from build123d import *

# Parameters (mm, degrees)
F0_W         = 52.4178380828
F0_H         = 38.1
F1_DEPTH     = 152.4
F3_DEPTH     = 152.401
F5_DEPTH     = 12.7
F7_DEPTH     = 19.05
F8_W         = 5.08
F8_H         = 2.54
F9_DEPTH     = 52.4188380828
F10_R        = 2.54
F11_T1_DEPTH = 18.199261314


# Not quite as in the source:
# - a fillet or chamfer that OpenCascade refuses, or shapes differently, is made with other operations: its cross-section is extruded or revolved along the edge and cut away or added


with BuildPart() as f1:
    # F0 (on Right) → F1 (new body)
    with BuildSketch(Plane.YZ):
        Rectangle(F0_W, F0_H)
    extrude(amount=-F1_DEPTH)

    # F2 (on face) → F3 (cut, through all)
    with BuildSketch(Plane.YZ):
        with BuildLine():
            Line((6.6756140975, -19.05), (10.4856140975, -19.05))
            Line((10.4856140975, -19.05), (10.4856140975, -2.54))
            ThreePointArc((10.4856140975, -2.54), (10.1136397096, -1.6419743879), (9.2156140975, -1.27))
            Line((9.2156140975, -1.27), (-9.2156140975, -1.27))
            ThreePointArc((-9.2156140975, -1.27), (-10.0011773128, -1.5421070023), (-10.4501149349, -2.241826087))
            Line((-10.4501149349, -2.241826087), (-13.6443859025, -15.4667596303))
            Line((-13.6443859025, -15.4667596303), (-9.9408833902, -16.3612813694))
            Line((-9.9408833902, -16.3612813694), (-7.2160704876, -5.08))
            Line((-7.2160704876, -5.08), (6.6756140975, -5.08))
            Line((6.6756140975, -5.08), (6.6756140975, -19.05))
        make_face()
    extrude(amount=-F3_DEPTH, mode=Mode.SUBTRACT)

    # F4 (on face) → F5 (cut)
    with BuildSketch(Plane.XY.offset(19.05)):
        Polygon((-142.875, -10.795), (-88.265, -10.795), (-88.265, -9.525), (0, -9.525), (0, 9.525), (-88.265, 9.525), (-88.265, 10.795), (-142.875, 10.795), (-142.875, 9.525), (-152.4, 9.525), (-152.4, -9.525), (-142.875, -9.525), align=None)
    extrude(amount=-F5_DEPTH, mode=Mode.SUBTRACT)

    # F6 (on face) → F7 (cut, through all)
    with BuildSketch(Plane.XZ.offset(-9.525)):
        Polygon((0, 6.35), (-33.02, 6.35), (-12.065, -19.05), (0, -19.05), align=None)
    extrude(amount=F7_DEPTH, mode=Mode.SUBTRACT)

    # F8 (on face) → F9 (cut, through all)
    with BuildSketch(Plane.XZ.offset(26.2089190414)):
        with Locations((-99.06, 1.27)):
            Rectangle(F8_W, F8_H)
        with Locations((-48.26, 1.27)):
            Rectangle(F8_W, F8_H)
    extrude(amount=-F9_DEPTH, mode=Mode.SUBTRACT)

    # F10
    f10_edges = [f1.edges().sort_by_distance(p)[0] for p in [
        (-87.995125, -7.21607, -5.08),
        (-87.995125, 6.675614, -5.08),
    ]]
    fillet(f10_edges, radius=F10_R)

    # F11: fillet of radius 2.54 on 2 edges, made by hand

    # F11_s2 → F11_t1 (cut)
    with BuildSketch(Plane.XY.offset(6.35)):
        with BuildLine():
            ThreePointArc((-86.0652954744, -9.525), (-87.3352954744, -9.8652954744), (-88.265, -10.795))
            Line((-88.265, -10.795), (-88.265, -9.525))
            Line((-88.265, -9.525), (-86.0652954744, -9.525))
        make_face()
        with BuildLine():
            ThreePointArc((-86.0652954744, 9.525), (-87.3352954744, 9.8652954744), (-88.265, 10.795))
            Line((-88.265, 10.795), (-88.265, 9.525))
            Line((-88.265, 9.525), (-86.0652954744, 9.525))
        make_face()
    extrude(amount=F11_T1_DEPTH, mode=Mode.SUBTRACT)


solid = f1.part
CAD build for the part. Positions are in the model's coordinates, mm. A direction names the side the tool comes from. Round coordinates to 2 decimals unless told otherwise and drop trailing zeros. Write each loop counter-clockwise with the first axis right and the second up, starting at its lowest first coordinate (ties: lowest second). Pieces come first, ordered by that corner, then holes. Notation, with made-up numbers: M 83,4 L 88,4 A16 ccw 88,27 Z; hole C 69.5,79.5 d3. An arc over 180 degrees is marked long. Use a Markdown table: item, result. Add a question column.
1. Slice it at A-A on y = 0. Give the number of separate pieces and of enclosed holes in the cut face, then the cut area to 3 significant figures.
2. Slice it at B-B on z = 12. Give the cut face in (x, y) (3 decimals), then the cut area to 3 significant figures.
3. Flat gauge pins, fed straight in: P1, Ø6.5, axis at x = -74, y = -5, coming from the +Z side; P2, Ø1.5, axis at x = -98.5, y = -5.5, coming from the +Z side; P3, Ø0.8, axis at y = -3.5, z = 1.5, coming from the +X side. Where does each tip first touch, or does it go through?
4. Slice it at D-D on x = -141.5. Give the cut face in (y, z) (3 decimals), then the cut area to 3 significant figures.
5. Slice it at C-C on z = -11. Give the cut face in (x, y).
6. Pull direction Y, two halves, no side cores. Call faces 4 (the face through (-42, 9.525, 11)), 5 (the face through (0, 18, 0)), 6 (the face through (-75, 26.209, 0)): released by +Y, released by -Y, zero draft, split by the parting line, or undercut.
7. 3-axis set-ups, long thin cutter, end or side, ignore diameter. For faces 1 (the face through (-75.13, -8.83, -11.76)), 2 (the face through (-116, -10.795, 13)), 3 (the face through (-17.908, -1.311, -11.967)): which of +Z, -Z, +X, -X, +Y, -Y reach the whole face in a straight line?
8. Drill centre lines: probe 1 along Y at (x, z) = (-120, 13) (3 decimals); probe 2 along Z at (x, y) = (-66, 3); probe 3 along Y at (x, z) = (-57.5, 12) (3 decimals). Where is each one in solid material? Low to high.
Reply:
| question | item | result |
|---|---|---|
| 1 | separate pieces | 2 |
| 1 | enclosed holes | 2 |
| 1 | area | 2,790 mm^2 |
| 2 | outline | M -152.4,-26.209 L 0,-26.209 L 0,-9.525 L -86.065,-9.525 A2.54 ccw -88.265,-10.795 L -142.875,-10.795 L -142.875,-9.525 L -152.4,-9.525 Z; M -152.4,9.525 L -142.875,9.525 L -142.875,10.795 L -88.265,10.795 A2.54 ccw -86.065,9.525 L 0,9.525 L 0,26.209 L -152.4,26.209 Z |
| 2 | area | 4,940 mm^2 |
| 3 | P1 | stops at z = 6.35 |
| 3 | P2 | stops at z = 6.35 |
| 3 | P3 | stops at x = -28.69 |
| 4 | outline | M -26.209,-19.05 L 6.676,-19.05 L 6.676,-7.62 A2.54 ccw 4.136,-5.08 L -5.217,-5.08 A2.54 ccw -7.686,-7.024 L -9.941,-16.361 L -13.644,-15.467 L -10.45,-2.242 A1.27 cw -9.216,-1.27 L 9.216,-1.27 A1.27 cw 10.486,-2.54 L 10.486,-19.05 L 26.209,-19.05 L 26.209,19.05 L 10.795,19.05 L 10.795,6.35 L -10.795,6.35 L -10.795,19.05 L -26.209,19.05 Z |
| 4 | area | 1,540 mm^2 |
| 5 | outline | M -152.4,-26.21 L 0,-26.21 L 0,-12.57 L -152.4,-12.57 Z; M -152.4,-8.65 L -18.71,-8.65 L -18.71,6.68 L -152.4,6.68 Z; M -152.4,10.49 L 0,10.49 L 0,26.21 L -152.4,26.21 Z |
| 6 | face 4 | undercut |
| 6 | face 5 | zero draft |
| 6 | face 6 | released by +Y |
| 7 | face 1 | +X, -X |
| 7 | face 2 | +Z |
| 7 | face 3 | +Z, +X |
| 8 | probe 1 | y = -26.209 to -10.795, 10.795 to 26.209 |
| 8 | probe 2 | z = -19.05 to -5.08, -1.27 to 6.35 |
| 8 | probe 3 | y = -26.209 to -9.525, 9.525 to 26.209 |
